from build123d import *

# Parameters (mm, degrees)
MAIN_DEPTH             = 17.5
SKETCH2_W              = 10.3
SKETCH2_H              = 28.5
HOLEFORSWITCH_DEPTH    = 31
SKETCH4_R              = 1.5
MAKERBEAMFIXHOLE_DEPTH = 22
HOLEFORTOOL_START      = -17
SKETCH5_R              = 4.25
HOLEFORTOOL_DEPTH      = 17


with BuildPart() as part:
    # Sketch1 → Main (new body, symmetric)
    with BuildSketch(Plane.XY):
        Polygon((-1, 26.45), (-1, 23.55), (0, 23.55), (0, 0), (20, 0), (20, 30), (0, 30), (0, 26.45), align=None)
    extrude(amount=MAIN_DEPTH, both=True)

    # Sketch2 → HoleForSwitch (cut, through all)
    with BuildSketch(Plane(origin=(0, 30, 0), x_dir=(1, 0, 0), z_dir=(0, 1, 0))):
        with Locations((10.85, 0)):
            Rectangle(SKETCH2_W, SKETCH2_H)
    extrude(amount=-HOLEFORSWITCH_DEPTH, mode=Mode.SUBTRACT)

    # Sketch4 → MakerBeamFixHole (cut, through all)
    with BuildSketch(Plane.ZY.offset(1)):
        with Locations((0, 25)):
            Circle(SKETCH4_R)
    extrude(amount=-MAKERBEAMFIXHOLE_DEPTH, mode=Mode.SUBTRACT)

    # Sketch5 → HoleForTool (cut)
    with BuildSketch(Plane(origin=(20, 0, 0), x_dir=(0, 0, -1), z_dir=(1, 0, 0)).offset(HOLEFORTOOL_START)):
        with Locations((0, 25)):
            Circle(SKETCH5_R)
    extrude(amount=HOLEFORTOOL_DEPTH, mode=Mode.SUBTRACT)


solid = part.part
Check sheet for the modelled part. Datum: model origin and axes. Units: mm. A direction names the side the tool comes from. Round coordinates to 2 decimals unless told otherwise and drop trailing zeros. Loops run counter-clockwise (first coordinate to the right, second up) from the corner with the lowest first, then second, coordinate; pieces in that order, holes last. Notation, with made-up numbers: M 25,28.25 L 58,28.25 A22 cw 58,46.25 Z; hole C -8.5,50.25 d11. An arc over 180 degrees is marked long. One line per item, written item: value.
(1) Thickness scan on line 1 (X direction, y = 25, z = -10.5); line 2 (Y direction, x = 18.8, z = 0); line 3 (X direction, y = 14.25, z = -7). Record the ranges inside material, lowest first.
Computed values:
line 1: x = -1 to 5.7, 16 to 20
line 2: y = 0 to 20.75, 29.25 to 30
line 3: x = 0 to 5.7, 16 to 20
(2) Sectioned sample at B-B, the plane y = 11.75. Record the cut outline in (x, z), then the cut area to 3 significant figures.
Computed values:
outline: M 0,-17.5 L 20,-17.5 L 20,17.5 L 0,17.5 Z; hole M 5.7,-14.25 L 16,-14.25 L 16,14.25 L 5.7,14.25 Z
area: 406 mm^2
(3) Release check for a two-part mould opening along X. For faces 1 (the face through (0, 12, 0)), 2 (the face through (16, 15, 0)), 3 (the face through (-0.5, 23.55, 9.1)) record: +X half, -X half, draft (parallel to the pull), parting line (faces both ways), or undercut.
Computed values:
face 1: -X half
face 2: undercut
face 3: draft
(4) Access from +Z, -Z, +X, -X, +Y, -Y to the whole of each face (thin tool, end or side, straight path). Record for faces 4 (the face through (-0.5, 23.55, -8.8)), 5 (the face through (0, 28, 0)), 6 (the face through (3, 25, -2)), 7 (the face through (11, 15, 14.25)).
Computed values:
face 4: +Z, -Z, -X, -Y
face 5: +Z, -Z, -X, +Y
face 6: +X
face 7: +Y, -Y
(5) Sectioned sample at D-D, the plane y = 25. Record the cut outline in (x, z).
Computed values:
outline: M -1,-17.5 L 20,-17.5 L 20,-4.25 L 16,-4.25 L 16,-14.25 L 5.7,-14.25 L 5.7,-4.25 L 3,-4.25 L 3,-1.5 L -1,-1.5 Z; M -1,1.5 L 3,1.5 L 3,4.25 L 5.7,4.25 L 5.7,14.25 L 16,14.25 L 16,4.25 L 20,4.25 L 20,17.5 L -1,17.5 Z
(6) Sectioned sample at A-A, the plane z = 10.5. Record the cut outline in (x, y), then the cut area to 3 significant figures.
Computed values:
outline: M -1,23.55 L 0,23.55 L 0,0 L 5.7,0 L 5.7,30 L 0,30 L 0,26.45 L -1,26.45 Z; M 16,0 L 20,0 L 20,30 L 16,30 Z
area: 294 mm^2
(7) Depth check by flat-ended pin: pin 1 Ø11 at (y, z) = (25, 0) entering from +X; pin 2 Ø5 at (x, z) = (8.5, 1.5) entering from +Y; pin 3 Ø1.1 at (y, z) = (28, 0.5) entering from -X; pin 4 Ø2.5 at (y, z) = (23, -1) entering from +X. Enter the tip coordinate at first touch or a pass-through.
Computed values:
pin 1: stops at x = 20
pin 2: passes through
pin 3: stops at x = 0
pin 4: stops at x = 3
(8) Sectioned sample at C-C, the plane x = 11.5. Record the cut outline in (y, z).
Computed values:
outline: M 0,-17.5 L 30,-17.5 L 30,-14.25 L 0,-14.25 Z; M 0,14.25 L 30,14.25 L 30,17.5 L 0,17.5 Z
